Source: CAD feature listing. Evaluate the final solid. Frame: model axes, mm. Face numbers are marked on the shaded views. A direction names the side the tool comes from. Give positions to 0.01 mm unless a question says otherwise; leave off trailing zeros. Order: outer loops, then holes, each group sorted by start corner. A loop starts at its lowest first (then second) coordinate and runs counter-clockwise, first axis right, second up. Notation, with made-up numbers: (-15.5, 77.5) -> (0.5, 77.5) arc R33 cw to (0.5, 108.5) -> close; hole circle Ø4 at (84, 22). An arc over 180 degrees is marked (long way). Answer in a Markdown table with one row per item.
```python
from build123d import *

# Parameters (mm, degrees)
SKETCH1_W           = 11
SKETCH1_H           = 5
SKETCH1_R           = 1
BOSS_EXTRUDE1_DEPTH = 2.6
SKETCH2_R           = 1.7
CUT_EXTRUDE1_DEPTH  = 1.5
FILLET1_R           = 1


with BuildPart() as part:
    # Sketch1 → Boss-Extrude1 (new body)
    with BuildSketch(Plane(origin=(0, 0, 0), x_dir=(1, 0, 0), z_dir=(0, 1, 0))):
        Rectangle(SKETCH1_W, SKETCH1_H)
        with Locations((-3.3, 0)):
            Circle(SKETCH1_R, mode=Mode.SUBTRACT)
        with Locations((3.3, 0)):
            Circle(SKETCH1_R, mode=Mode.SUBTRACT)
    extrude(amount=BOSS_EXTRUDE1_DEPTH)

    # Sketch2 → Cut-Extrude1 (cut)
    with BuildSketch(Plane(origin=(0, 2.6, 0), x_dir=(1, 0, 0), z_dir=(0, 1, 0))):
        with Locations((-3.3, 0)):
            Circle(SKETCH2_R)
        with Locations((3.3, 0)):
            Circle(SKETCH2_R)
    extrude(amount=-CUT_EXTRUDE1_DEPTH, mode=Mode.SUBTRACT)

    # Fillet1
    fillet1_edges = [part.edges().sort_by_distance(p)[0] for p in [
        (5.5, 1.3, 2.5),
        (-5.5, 1.3, 2.5),
        (-5.5, 1.3, -2.5),
        (5.5, 1.3, -2.5),
    ]]
    fillet(fillet1_edges, radius=FILLET1_R)


solid = part.part
```
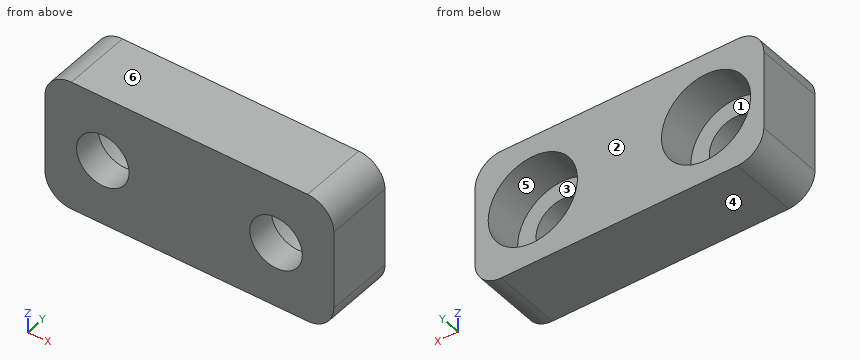
(1) Access query for the marked faces 1 and 2. Directions: +Z, -Z, +X, -X, +Y, -Y. A direction counts if a zero-diameter tool reaches every point of the face in a straight line with its end or side. Return the directions, or none.
A:
| item | result |
|---|---|
| face 1 | +Y |
| face 2 | +Z, -Z, +X, -X, +Y |
(2) Section query D-D (y = 1.75). Return the cut outline in (x, z), plus the area to 3 significant figures.
A:
| item | result |
|---|---|
| outline | (-5.5, -1.5) arc R1 ccw to (-4.5, -2.5) -> (4.5, -2.5) arc R1 ccw to (5.5, -1.5) -> (5.5, 1.5) arc R1 ccw to (4.5, 2.5) -> (-4.5, 2.5) arc R1 ccw to (-5.5, 1.5) -> close; hole circle Ø3.4 at (-3.3, 0); hole circle Ø3.4 at (3.3, 0) |
| area | 36.0 mm^2 |
(3) Pull-direction query (Z, two-part tool) for the marked faces 3, 4, 5 and 6; classes: +Z half, -Z half, draft (parallel to the pull), parting line (faces both ways), or undercut.
A:
| item | result |
|---|---|
| face 3 | undercut |
| face 4 | -Z half |
| face 5 | undercut |
| face 6 | +Z half |
(4) Ray query, probe 1 along X at (y, z) = (2.05, -0.1); probe 2 along Z at (x, y) = (3.3, 1.5); probe 3 along X at (y, z) = (0.4, 0). Return the intervals inside material, ascending.
A:
| item | result |
|---|---|
| probe 1 | x = -5.5 to -5, -1.6 to 1.6, 5 to 5.5 |
| probe 2 | z = -2.5 to -1.7, 1.7 to 2.5 |
| probe 3 | x = -5.5 to -4.3, -2.3 to 2.3, 4.3 to 5.5 |
(5) First-contact query: pin 1 Ø2.5 at (x, z) = (3.3, 0) entering from +Y. Flat tip, straight axial feed; report the tip coordinate or a pass-through.
A:
| item | result |
|---|---|
| pin 1 | stops at y = 1.1 |
(6) Section query C-C (z = -0.8). Return the cut outline in (x, y), plus the area to 3 significant figures.
A:
| item | result |
|---|---|
| outline | (-5.5, 0) -> (-3.9, 0) -> (-3.9, 1.1) -> (-4.8, 1.1) -> (-4.8, 2.6) -> (-5.5, 2.6) -> close; (-2.7, 0) -> (2.7, 0) -> (2.7, 1.1) -> (1.8, 1.1) -> (1.8, 2.6) -> (-1.8, 2.6) -> (-1.8, 1.1) -> (-2.7, 1.1) -> close; (3.9, 0) -> (5.5, 0) -> (5.5, 2.6) -> (4.8, 2.6) -> (4.8, 1.1) -> (3.9, 1.1) -> close |
| area | 17.0 mm^2 |
(7) Section query A-A (y = 0.4). Return the cut outline in (x, z), plus the area to 3 significant figures.
A:
| item | result |
|---|---|
| outline | (-5.5, -1.5) arc R1 ccw to (-4.5, -2.5) -> (4.5, -2.5) arc R1 ccw to (5.5, -1.5) -> (5.5, 1.5) arc R1 ccw to (4.5, 2.5) -> (-4.5, 2.5) arc R1 ccw to (-5.5, 1.5) -> close; hole circle Ø2 at (-3.3, 0); hole circle Ø2 at (3.3, 0) |
| area | 47.9 mm^2 |
(8) Section query B-B (x = -3.3). Return the cut outline in (y, z).
A:
| item | result |
|---|---|
| outline | (0, -2.5) -> (2.6, -2.5) -> (2.6, -1.7) -> (1.1, -1.7) -> (1.1, -1) -> (0, -1) -> close; (0, 1) -> (1.1, 1) -> (1.1, 1.7) -> (2.6, 1.7) -> (2.6, 2.5) -> (0, 2.5) -> close |
